Here's how the part is built. I have some questions about the finished solid (model axes, mm). A direction names the side the tool comes from. Round coordinates to 2 decimals unless told otherwise and drop trailing zeros. Loops run counter-clockwise (first coordinate to the right, second up) from the corner with the lowest first, then second, coordinate; pieces in that order, holes last. Notation, with made-up numbers: M 73,-21 L 101,-21 A34 ccw 101,9 Z; hole C 9.25,24 d9. An arc over 180 degrees is marked long. Answer as a JSON object with one key per item and string values.
Autodesk Inventor part; units mm, degrees
ref_plane "YZ Plane" through (0, 0, 0) normal (1, 0, 0) x (0, 1, 0)
ref_plane "XZ Plane" through (0, 0, 0) normal (0, 1, 0) x (-1, 0, 0)
ref_plane "XY Plane" through (0, 0, 0) normal (0, 0, 1) x (1, 0, 0)
sketch "Block1" plane through (0, 0, 0) normal (0, 0, 1) x (1, 0, 0)
  circle A0 centre (74.029, 24.2723) radius 1
  line L0 (49.279, 30.4723) -> (71.779, 30.4723)
  line L1 (71.779, 30.4723) -> (71.779, 18.0723)
  line L2 (71.779, 18.0723) -> (49.279, 18.0723)
  line L3 (49.279, 18.0723) -> (49.279, 30.4723)
  line L4 (49.279, 30.4723) -> (44.779, 30.4723)
  line L5 (44.779, 30.4723) -> (44.779, 18.0723)
  line L6 (44.779, 18.0723) -> (49.279, 18.0723)
  line L7 (49.279, 18.0723) -> (49.279, 30.4723)
  line L8 (71.779, 30.4723) -> (76.279, 30.4723)
  line L9 (76.279, 30.4723) -> (76.279, 18.0723)
  line L10 (76.279, 18.0723) -> (71.779, 18.0723)
  line L11 (71.779, 18.0723) -> (71.779, 30.4723)
  line L12 (44.779, 24.2723) -> (76.279, 24.2723) construction
  line L13 (47.029, 30.4723) -> (47.029, 18.0723) construction
  circle A1 centre (47.029, 24.2723) radius 1
  line L14 (74.029, 30.4723) -> (74.029, 18.0723) construction
  point P0 (60.979, 24.0984)
  dimension "d22" = 22.5
  dimension "d23" = 12.4
  dimension "d24" = 4.5
  dimension "d25" = 4.5
  dimension "d26" = 2
  dimension "d27" = 2
sketch "Sketch1" plane through (0, 0, 0) normal (0, 0, 1) x (1, 0, 0)
  line L0 (-92.7646, -8.503) -> (-89.7646, -8.503)
  line L1 (-89.7646, -8.503) -> (-89.7646, -11.753)
  line L2 (-89.7646, -11.753) -> (-92.7646, -11.753)
  line L3 (-92.7646, -11.753) -> (-92.7646, -8.503)
  line L4 (-92.7646, -21.6527) -> (-89.7646, -21.6527)
  line L5 (-89.7646, -21.6527) -> (-89.7646, -21.7527)
  line L6 (-89.7646, -21.7527) -> (-92.7646, -21.7527)
  line L7 (-92.7646, -21.7527) -> (-92.7646, -21.6527)
  line L8 (-39.1148, 14.5179) -> (-15.1148, 14.5179)
  line L9 (-15.1148, 14.5179) -> (-15.1148, 18.7679)
  line L10 (-15.1148, 18.7679) -> (-39.1148, 18.7679)
  line L11 (-39.1148, 18.7679) -> (-39.1148, 14.5179)
  line L12 (-34.1148, 22.0179) -> (-20.1148, 22.0179)
  line L13 (-20.1148, 22.0179) -> (-20.1148, 18.7679)
  line L14 (-20.1148, 18.7679) -> (-34.1148, 18.7679)
  line L15 (-34.1148, 18.7679) -> (-34.1148, 22.0179)
  line L16 (-39.1148, 16.6429) -> (-15.1148, 16.6429) construction
  line L17 (-27.1148, 22.0179) -> (-27.1148, 18.7679) construction
  line L18 (-27.1148, 18.7679) -> (-27.1148, 14.5179) construction
  line L19 (-34.1148, 11.2679) -> (-20.1148, 11.2679)
  line L20 (-20.1148, 11.2679) -> (-20.1148, 14.5179)
  line L21 (-20.1148, 14.5179) -> (-34.1148, 14.5179)
  line L22 (-34.1148, 14.5179) -> (-34.1148, 11.2679)
  line L23 (-27.1148, 11.2679) -> (-27.1148, 14.5179) construction
  point P0 (0, 0)
  point P1 (-27.1148, 14.5179)
  dimension "d3" = 3
  dimension "mat" = 3.25
  dimension "d5" = 3
  dimension "kerf" = 0.1
  dimension "d42" = 24
  dimension "d43" = 4.25
  dimension "d44" = 14
  dimension "d45" = 3.25
extrude "Extrusion6" add sketch "Sketch1" along normal blind 3.25 contours L11 L10 L9 L8 | L8 L20 L19 L22 | L15 L12 L13 L10
equation "\"d45\" = mat"
equation "\"d46\" = mat"
properties part number "body-back"
Item 1: For P1, Ø1, axis at x = -36.5, z = 2, coming from the -Y side; P2, Ø2, axis at x = -25, y = 20, coming from the -Z side; P3, Ø1, axis at x = -37.5, z = 1.5, coming from the +Y side; P4, Ø1, axis at y = 20, z = 2, coming from the -X side, each with a flat end and sliding along its axis, tell me the tip position at first contact or that it passes through.
Solution:
{"P1": "stops at y = 14.52", "P2": "stops at z = 0", "P3": "stops at y = 18.77", "P4": "stops at x = -34.11"}
Item 2: I want a section at A-A on z = 0.6. List the corners of the cut face in (x, y) for me.
Solution:
{"outline": "M -39.11,14.52 L -34.11,14.52 L -34.11,11.27 L -20.11,11.27 L -20.11,14.52 L -15.11,14.52 L -15.11,18.77 L -20.11,18.77 L -20.11,22.02 L -34.11,22.02 L -34.11,18.77 L -39.11,18.77 Z"}
Item 3: I want a section at C-C on y = 20.25. List the corners of the cut face in (x, z) for me, plus the area to 3 significant figures.
Solution:
{"outline": "M -34.11,0 L -20.11,0 L -20.11,3.25 L -34.11,3.25 Z", "area": "45.5 mm2"}
Item 4: I want a section at B-B on x = -17.25. List the corners of the cut face in (y, z) for me, plus the area to 3 significant figures.
Solution:
{"outline": "M 14.52,0 L 18.77,0 L 18.77,3.25 L 14.52,3.25 Z", "area": "13.8 mm2"}
Item 5: For faces 1 (the face through (-34.115, 13, 2)), 2 (the face through (-34.115, 20, 2)), 3 (the face through (-20.115, 13, 2)), which set-ups out of +Z, -Z, +X, -X, +Y, -Y let a thin tool reach every point of the face, with its end or its side?
Solution:
{"face 1": "+Z, -Z, -X, -Y", "face 2": "+Z, -Z, -X, +Y", "face 3": "+Z, -Z, +X, -Y"}
Item 6: If I drill on L1, parallel to Y at x = -38, z = 0.55; L2, parallel to X at y = 14.25, z = 2.35, over which ranges is the centre line in solid material (lowest first)? Write a range as from..to.
Solution:
{"L1": "y = 14.52..18.77", "L2": "x = -34.11..-20.11"}
